Part model, mm, in its own coordinate system. Round coordinates to 2 decimals unless told otherwise and drop trailing zeros. Loops run counter-clockwise (first coordinate to the right, second up) from the corner with the lowest first, then second, coordinate; pieces in that order, holes last. Notation, with made-up numbers: (63, 21.5) - (91, 21.5) arc R34 ccw to (91, 56.5) - close; hole circle Ø4 at (62, -38.5). An arc over 180 degrees is marked (long way). Put each result on its own line as item: value.
from build123d import *

# Parameters (mm, degrees)
F1_DEPTH = 1


with BuildPart() as f1:
    # F0 (on Top) → F1 (new body)
    with BuildSketch(Plane.XY):
        with BuildLine():
            ThreePointArc((0.235507, 1.058424), (0.971203, 0.284898), (2, 0))
            Line((2, 0), (63, 0))
            Line((63, 0), (63, 26))
            ThreePointArc((63, 26), (62.414214, 27.414214), (61, 28))
            Line((61, 28), (2, 28))
            ThreePointArc((2, 28), (0.971203, 27.715102), (0.235507, 26.941576))
            ThreePointArc((0.235507, 26.941576), (4.85153, 21.189024), (6.5, 14))
            ThreePointArc((6.5, 14), (4.85153, 6.810976), (0.235507, 1.058424))
        make_face()
    extrude(amount=F1_DEPTH)


solid = f1.part
1. Band-saw the part on C-C (y = 19.25). List the corners of the cut face in (x, z).
A:
outline: (5.64, 0) - (63, 0) - (63, 1) - (5.64, 1) - close
2. Probe line 1 along X through (y, z) = (14, 0.75); line 2 along X through (y, z) = (1.25, 0.9). List the from-to ranges inside material, lowest first. Write a range as [from, to].
A:
line 1: x = [6.5, 63]
line 2: x = [0.47, 63]
3. Band-saw the part on A-A (z = 0.4). List the corners of the cut face in (x, y).
A:
outline: (0.24, 1.06) arc R2 ccw to (2, 0) - (63, 0) - (63, 26) arc R2 ccw to (61, 28) - (2, 28) arc R2 ccw to (0.24, 26.94) arc R16.5 cw to (6.5, 14) arc R16.5 cw to start
4. Band-saw the part on B-B (y = 22.75). List the corners of the cut face in (x, z), plus the area to 3 significant figures.
A:
outline: (3.99, 0) - (63, 0) - (63, 1) - (3.99, 1) - close
area: 59.0 mm²
